```python
from build123d import *

# Parameters (mm, degrees)
SKETCH_2_R               = 0.7
CUT_EXTRUDE_1_DEPTH      = 5.5
CUT_EXTRUDE_1_DEPTH_BACK = 5.5
CHAMFER_1_SIZE           = 1


with BuildPart() as part:
    # 草图1 → 旋转1 (revolve)
    with BuildSketch(Plane(origin=(0, 0, 0), x_dir=(1, 0, 0), z_dir=(0, 1, 0))):
        Polygon((0, 0), (-3, 0), (-3, 44), (-2, 44), (-2, 45), (-4.5, 45), (-4.5, 47), (0, 47), align=None)
    revolve(axis=Axis((0, 0, -47), (0, 0, 1)))

    # 草图2 → 切除-拉伸1 (cut, two sides)
    with BuildSketch(Plane(origin=(0, 0, 0), x_dir=(1, 0, 0), z_dir=(0, 1, 0))) as cut_extrude_1_sk:
        with Locations((0, 2.5)):
            Circle(SKETCH_2_R)
    extrude(amount=CUT_EXTRUDE_1_DEPTH, mode=Mode.SUBTRACT)
    extrude(cut_extrude_1_sk.sketch, amount=-CUT_EXTRUDE_1_DEPTH_BACK, mode=Mode.SUBTRACT)

    # 倒角1
    chamfer_1_edges = [part.edges().sort_by_distance(p)[0] for p in [
        (4.5, 0, -47),
        (3, 0, 0),
    ]]
    chamfer(chamfer_1_edges, length=CHAMFER_1_SIZE)


solid = part.part
```
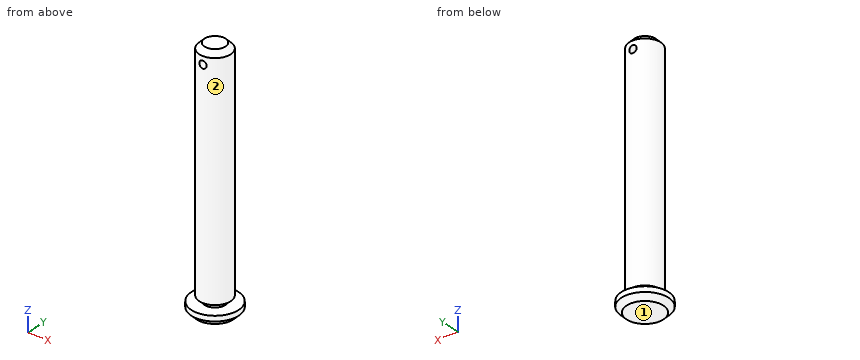
The listing builds one solid part. Answer for the finished solid, in the listing's coordinates (mm). Face numbers are marked on the shaded views. A direction names the side the tool comes from. Coordinates: 2 decimals unless noted, no trailing zeros. Loops run counter-clockwise (first coordinate to the right, second up) from the corner with the lowest first, then second, coordinate; pieces in that order, holes last. Notation, with made-up numbers: (61, 65) - (72, 65) arc R23 ccw to (72, 73) - close; hole circle Ø2 at (17, 88). An arc over 180 degrees is marked (long way). Use a Markdown table: item, result. Add a question column.
1) Given pin 1 (2 mm diameter, centred on x = 1.5, y = -3.5, fed in from +Z); pin 2 (4.5 mm diameter, centred on x = -0.5, y = -2, fed in from +Z); pin 3 (2 mm diameter, centred on x = 0, z = -2.5, fed in from -Y), each flat-ended and moving along its own axis, determine where each tip first touches the part or whether it passes through.
2) The part is cut by section C-C, the plane z = -2.5. Give the vertices of the cut face in (x, y), and give its area (3 significant figures).
3) Find the intervals of material crossed by line 1 (Z direction, x = 0, y = -1.5); line 2 (X direction, y = 0, z = -2.5); line 3 (X direction, y = 1.75, z = -2.5), in increasing order.
4) The part is cut by section A-A, the plane x = 0. Give the vertices of the cut face in (y, z), and give its area (3 significant figures).
5) For the marked faces 1 and 2, determine the directions among +Z, -Z, +X, -X, +Y, -Y from which every point of the face is accessible in a straight line to the end or side of a thin tool.
6) The part is cut by section B-B, the plane y = 0. Give the vertices of the cut face in (x, z).
7) The part is cut by section D-D, the plane z = -30. Give the vertices of the cut face in (x, y), and give its area (3 significant figures).
Here are the results:
| question | item | result |
|---|---|---|
| 1 | pin 1 | stops at z = -0.81 |
| 1 | pin 2 | stops at z = 0 |
| 1 | pin 3 | stops at y = -3 |
| 2 | outline | (-0.7, -2.92) - (-0.7, 2.92) arc R3 ccw to start; (0.7, -2.92) arc R3 ccw to (0.7, 2.92) - close |
| 2 | area | 20.0 mm^2 |
| 3 | line 1 | z = -47 to -3.2, -1.8 to 0 |
| 3 | line 2 | x = -3 to -0.7, 0.7 to 3 |
| 3 | line 3 | x = -2.44 to -0.7, 0.7 to 2.44 |
| 4 | outline | (-4.5, -46) - (-3.5, -47) - (3.5, -47) - (4.5, -46) - (4.5, -45) - (2, -45) - (2, -44) - (3, -44) - (3, -3.2) - (-3, -3.2) - (-3, -44) - (-2, -44) - (-2, -45) - (-4.5, -45) - close; (-3, -1.8) - (3, -1.8) - (3, -1) - (2, 0) - (-2, 0) - (-3, -1) - close |
| 4 | area | 276 mm^2 |
| 5 | face 1 | -Z, +X, -X, +Y, -Y |
| 5 | face 2 | +Z |
| 6 | outline | (-4.5, -46) - (-3.5, -47) - (3.5, -47) - (4.5, -46) - (4.5, -45) - (2, -45) - (2, -44) - (3, -44) - (3, -1) - (2, 0) - (-2, 0) - (-3, -1) - (-3, -44) - (-2, -44) - (-2, -45) - (-4.5, -45) - close; hole circle Ø1.4 at (0, -2.5) |
| 7 | outline | circle Ø6 at (0, 0) |
| 7 | area | 28.3 mm^2 |
